```python
from build123d import *

# Parameters (mm, degrees)
BOSS_EXTRUDE1_DEPTH     = 3.175
FILLET1_R               = 3.175
CUT_EXTRUDE1_DEPTH      = 192.340110238
CUT_EXTRUDE1_DEPTH_BACK = 192.340110238
FILLET2_R               = 6.35


with BuildPart() as part:
    # Sketch1 → Boss-Extrude1 (new body)
    with BuildSketch(Plane.XY):
        Polygon((-19.84375, 0), (0, 9.525), (19.84375, 0), (152.4, 121.92), (-152.4, 121.92), align=None)
    extrude(amount=BOSS_EXTRUDE1_DEPTH)

    # Fillet1
    fillet1_edges = [part.edges().sort_by_distance(p)[0] for p in [
        (0, 9.525, 1.5875),
        (-19.84375, 0, 1.5875),
        (-152.4, 121.92, 1.5875),
        (152.4, 121.92, 1.5875),
        (19.84375, 0, 1.5875),
    ]]
    fillet(fillet1_edges, radius=FILLET1_R)

    # Sketch2 → Cut-Extrude1 (cut, two sides: drawn at the far end of the back side and taken through both)
    with BuildSketch(Plane.XY.offset(3.175).offset(-CUT_EXTRUDE1_DEPTH_BACK)):
        Polygon((-82.940049134, 62.347230555), (-22.177311492, 118.745), (-144.257936486, 118.745), align=None)
        Polygon((-19.84375, 4.313748238), (-19.84375, 116.579072853), (-80.595875999, 60.191152749), align=None)
        with BuildLine():
            Line((16.66875, 5.045817854), (16.66875, 118.745))
            Line((16.66875, 118.745), (-16.66875, 118.745))
            Line((-16.66875, 118.745), (-16.66875, 5.045817854))
            Line((-16.66875, 5.045817854), (-2.747842279, 11.72785356))
            ThreePointArc((-2.747842279, 11.72785356), (0, 12.353182146), (2.747842279, 11.72785356))
            Line((2.747842279, 11.72785356), (16.66875, 5.045817854))
        make_face()
        Polygon((80.595875999, 60.191152749), (19.84375, 116.579072853), (19.84375, 4.313748238), align=None)
        Polygon((144.257936486, 118.745), (22.177311492, 118.745), (82.940049134, 62.347230555), align=None)
    extrude(amount=CUT_EXTRUDE1_DEPTH + CUT_EXTRUDE1_DEPTH_BACK, mode=Mode.SUBTRACT)

    # Fillet2
    fillet2_edges = [part.edges().sort_by_distance(p)[0] for p in [
        (-22.177311492, 118.745, 1.5875),
        (-82.940049134, 62.347230555, 1.5875),
        (-144.257936486, 118.745, 1.5875),
        (19.84375, 116.579072853, 1.5875),
        (80.595875999, 60.191152749, 1.5875),
        (19.84375, 4.313748238, 1.5875),
        (22.177311492, 118.745, 1.5875),
        (144.257936486, 118.745, 1.5875),
        (82.940049134, 62.347230555, 1.5875),
        (-16.66875, 5.045817854, 1.5875),
        (-16.66875, 118.745, 1.5875),
        (16.66875, 118.745, 1.5875),
        (16.66875, 5.045817854, 1.5875),
        (-19.84375, 116.579072853, 1.5875),
        (-19.84375, 4.313748238, 1.5875),
        (-80.595875999, 60.191152749, 1.5875),
    ]]
    fillet(fillet2_edges, radius=FILLET2_R)


solid = part.part
```
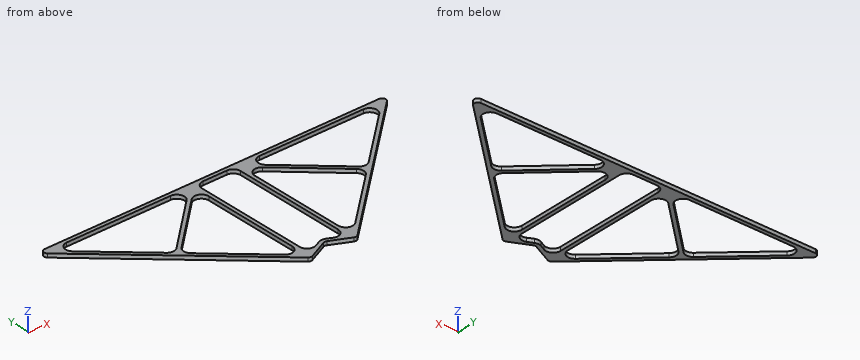
Work out the finished part from the listing and answer in its coordinate system (mm). Coordinates: 2 decimals unless noted, no trailing zeros. Loops run counter-clockwise (first coordinate to the right, second up) from the corner with the lowest first, then second, coordinate; pieces in that order, holes last. Notation, with made-up numbers: (-14, -24.5) - (-7, -24.5) arc R17 cw to (-7, -13.5) - close; hole circle Ø2 at (57.5, -22). An arc over 180 degrees is marked (long way). Use a Markdown table: item, result.
Item 1: Find section C-C, the plane z = 1.6. State how many separate pieces and enclosed holes the cut face has, and give its area (3 significant figures).
Evaluation:
| item | result |
|---|---|
| separate pieces | 1 |
| enclosed holes | 5 |
| area | 3,920 mm2 |
Item 2: Given pin 1 Ø1 at (x, z) = (-53, 2) entering from -Y; pin 2 Ø1 at (x, z) = (-65.5, 1) entering from -Y; pin 3 Ø1.6 at (y, z) = (78.5, 1.5) entering from +X, each flat-ended and moving along its own axis, determine where each tip first touches the part or whether it passes through.
Evaluation:
| item | result |
|---|---|
| pin 1 | stops at y = 30.04 |
| pin 2 | stops at y = 41.53 |
| pin 3 | stops at x = 106.06 |
Item 3: Find section A-A, the plane y = 84. Determine the outline of the cut face in (x, z) (3 decimals), and give its area (3 significant figures).
Evaluation:
| item | result |
|---|---|
| outline | (-111.172, 0) - (-106.482, 0) - (-106.482, 3.175) - (-111.172, 3.175) - close; (-59.611, 0) - (-54.944, 0) - (-54.944, 3.175) - (-59.611, 3.175) - close; (-19.844, 0) - (-16.669, 0) - (-16.669, 3.175) - (-19.844, 3.175) - close; (16.669, 0) - (19.844, 0) - (19.844, 3.175) - (16.669, 3.175) - close; (54.944, 0) - (59.611, 0) - (59.611, 3.175) - (54.944, 3.175) - close; (106.482, 0) - (111.172, 0) - (111.172, 3.175) - (106.482, 3.175) - close |
| area | 79.6 mm2 |
Item 4: Find section B-B, the plane x = -122.5. Determine the outline of the cut face in (y, z) (3 decimals), and give its area (3 significant figures).
Evaluation:
| item | result |
|---|---|
| outline | (94.419, 0) - (98.733, 0) - (98.733, 3.175) - (94.419, 3.175) - close; (118.745, 0) - (121.92, 0) - (121.92, 3.175) - (118.745, 3.175) - close |
| area | 23.8 mm2 |
Item 5: Consider probe 1 along X at (y, z) = (55.5, 2.05); probe 2 along Y at (x, z) = (-48, 1.45) (3 decimals); probe 3 along X at (y, z) = (73, 0.45). Determine where each line is inside the solid, lowest interval first. Write a range as from..to.
Evaluation:
| item | result |
|---|---|
| probe 1 | x = -80.19..-75.5, -19.84..-16.67, 16.67..19.84, 75.5..80.19 |
| probe 2 | y = 25.897..30.211, 90.445..94.777, 118.745..121.92 |
| probe 3 | x = -99.21..-94.52, -71.46..-66.8, -19.84..-16.67, 16.67..19.84, 66.8..71.46, 94.52..99.21 |
Item 6: Find section D-D, the plane x = -58.5. Determine the outline of the cut face in (y, z) (1 decimal).
Evaluation:
| item | result |
|---|---|
| outline | (35.6, 0) - (39.9, 0) - (39.9, 3.2) - (35.6, 3.2) - close; (80.7, 0) - (85, 0) - (85, 3.2) - (80.7, 3.2) - close; (118.7, 0) - (121.9, 0) - (121.9, 3.2) - (118.7, 3.2) - close |
